```python
from build123d import *

# Parameters (mm, degrees)
F0_R     = 10
F1_DEPTH = 10
F2_R     = 10
F3_R     = 10
F5_DEPTH = 5
F6_R     = 5
F7_R     = 5
F8_R     = 2


with BuildPart() as f1:
    # F0 (on Front) → F1 (new body, symmetric)
    with BuildSketch(Plane.XZ):
        with BuildLine():
            ThreePointArc((-36.194757, 10.609343), (-32.603742, 5.835876), (-31.329407, 0))
            Line((-31.329407, 0), (40.670593, 0))
            ThreePointArc((40.670593, 0), (42.681766, 9.617248), (48.378215, 17.622667))
            Line((48.378215, 17.622667), (-36.194757, 10.609343))
        make_face()
        with BuildLine():
            Line((40.670593, 0), (-31.329407, 0))
            ThreePointArc((-31.329407, 0), (-32.603742, -5.835876), (-36.194757, -10.609343))
            Line((-36.194757, -10.609343), (48.378215, -17.622667))
            ThreePointArc((48.378215, -17.622667), (42.681766, -9.617248), (40.670593, 0))
        make_face()
        with BuildLine():
            ThreePointArc((48.378215, 17.622667), (42.681766, 9.617248), (40.670593, 0))
            ThreePointArc((40.670593, 0), (42.681766, -9.617248), (48.378215, -17.622667))
            ThreePointArc((48.378215, -17.622667), (74.287841, -21.988828), (88.670593, 0))
            ThreePointArc((88.670593, 0), (74.287841, 21.988828), (48.378215, 17.622667))
        make_face()
        with BuildLine():
            ThreePointArc((82.670593, 0), (64.670593, -18), (46.670593, 0))
            ThreePointArc((46.670593, 0), (64.670593, 18), (82.670593, 0))
        make_face(mode=Mode.SUBTRACT)
        with BuildLine():
            ThreePointArc((-36.194757, -10.609343), (-32.603742, -5.835876), (-31.329407, 0))
            ThreePointArc((-31.329407, 0), (-32.603742, 5.835876), (-36.194757, 10.609343))
            ThreePointArc((-36.194757, 10.609343), (-59.329407, 0), (-36.194757, -10.609343))
        make_face()
        with Locations((-45.329407, 0)):
            Circle(F0_R, mode=Mode.SUBTRACT)
    extrude(amount=F1_DEPTH, both=True)

    # F2
    f2_edges = [f1.edges().sort_by_distance(p)[0] for p in [
        (-36.194757, 0, 10.609343),
    ]]
    fillet(f2_edges, radius=F2_R)

    # F3
    f3_edges = [f1.edges().sort_by_distance(p)[0] for p in [
        (48.378215, 5, 17.622667),
        (48.378215, 5, -17.622667),
        (-36.194757, 0, -10.609343),
    ]]
    fillet(f3_edges, radius=F3_R)

    # F4 (on face) → F5 (cut)
    with BuildSketch(Plane.XZ.offset(10)):
        Polygon((42.828392, 13.610834), (-33.350925, 8.230139), (-33.350925, -8.230139), (42.828392, -13.610834), align=None)
    extrude(amount=-F5_DEPTH, mode=Mode.SUBTRACT)

    # F6
    f6_edges = [f1.edges().sort_by_distance(p)[0] for p in [
        (-33.350925, -7.5, 8.230139),
        (-33.350925, -7.5, -8.230139),
    ]]
    fillet(f6_edges, radius=F6_R)

    # F7
    f7_edges = [f1.edges().sort_by_distance(p)[0] for p in [
        (42.828392, -7.5, 13.610834),
        (42.828392, -7.5, -13.610834),
    ]]
    fillet(f7_edges, radius=F7_R)

    # F8
    f8_edges = [f1.edges().sort_by_distance(p)[0] for p in [
        (4.386452, -5, 10.895604),
        (-55.329407, -10, 0),
    ]]
    fillet(f8_edges, radius=F8_R)


solid = f1.part
```
Input: part model. Units: mm. Frame: model coordinates. A direction names the side the tool comes from. Give positions to 0.01 mm unless a question says otherwise; leave off trailing zeros. Order: outer loops, then holes, each group sorted by start corner. A loop starts at its lowest first (then second) coordinate and runs counter-clockwise, first axis right, second up. Notation, with made-up numbers: (88, 64.25) - (111, 64.25) arc R13 ccw to (111, 75.25) - close; hole circle Ø11 at (78, 48.5). An arc over 180 degrees is marked (long way). One line per item, written item: value.
1. Reachability of faces 1 (the face through (3.96, -5.6, 10.29)), 2 (the face through (5.77, -0.14, -14.09)), 3 (the face through (31, -10, -14)) from +Z, -Z, +X, -X, +Y, -Y: full face, straight path, thin tool, end or side. Return the list, or none.
Determined:
face 1: -Y
face 2: -Z, +Y, -Y
face 3: +Z, -Z, +X, -X, -Y
2. Pin query (flat end, axial travel): pin 1 Ø1 at (y, z) = (-3.5, 10) entering from -X; pin 2 Ø1 at (x, y) = (-18, 6.5) entering from -Z; pin 3 Ø2 at (x, y) = (35, -1) entering from -Z; pin 4 Ø24.5 at (x, z) = (13, 2) entering from -Y. Return the tip coordinate at first contact, or that it passes through.
Determined:
pin 1: x = -55.61
pin 2: z = -12.16
pin 3: z = -16.6
pin 4: y = -10
3. Line query: probe 1 along X at (y, z) = (-4.5, -1.5); probe 2 along Z at (x, y) = (65, 2); probe 3 along X at (y, z) = (1, 5). Output: solid intervals per line, ascending.
Determined:
probe 1: -59.25 to -55.22, -35.44 to 46.73, 82.61 to 88.62
probe 2: -24 to -18, 18 to 24
probe 3: -58.41 to -53.99, -36.67 to 47.38, 81.96 to 88.14
4. Cut plane A-A, the plane y = -2.5. Output: boundary loops of the cut face in (x, z).
Determined:
outline: (-38.42, -12.17) arc R10 cw to (-32.65, -10.9) - (45.27, -17.37) arc R10 cw to (50.39, -19.29) arc R24 ccw to (88.67, 0) arc R24 ccw to (50.39, 19.29) arc R10 cw to (45.27, 17.37) - (-32.65, 10.9) arc R10 cw to (-38.42, 12.17) arc R14 ccw (long way) to start; hole circle Ø20 at (-45.33, 0); hole circle Ø36 at (64.67, 0)
5. Draft query along X for faces 4 (the face through (47.932, 0.14, 17.958)), 5 (the face through (41.195, -8.479, -11.942)), 6 (the face through (14, 10, 0)), 7 (the face through (3.923, -8.521, -10.863)). Return one class per face: released by +X, released by -X, zero draft, split by the parting line, or undercut.
Determined:
face 4: released by -X
face 5: undercut
face 6: zero draft
face 7: undercut
6. Cut plane B-B, the plane x = 70. Output: boundary loops of the cut face in (y, z), and give its area (3 significant figures).
Determined:
outline: (-10, -23.4) - (10, -23.4) - (10, -17.19) - (-10, -17.19) - close; (-10, 17.19) - (10, 17.19) - (10, 23.4) - (-10, 23.4) - close
area: 248 mm2
